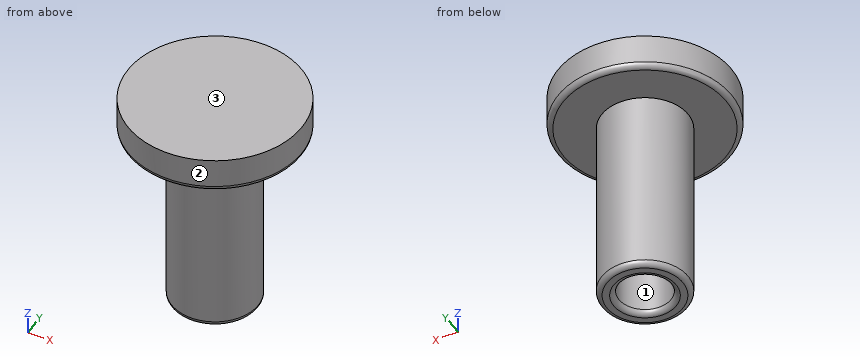
from build123d import *

# Parameters (mm, degrees)
F0_R     = 4.99
F1_DEPTH = 2
F2_R     = 2.485
F3_DEPTH = 11
F4_R     = 1.5
F5_DEPTH = 5
F6_R     = 0.3


with BuildPart() as f1:
    # F0 (on Top) → F1 (new body)
    with BuildSketch(Plane.XY):
        Circle(F0_R)
    extrude(amount=F1_DEPTH)

    # F2 (on face) → F3 (join)
    with BuildSketch(Plane(origin=(0, 0, 0), x_dir=(1, 0, 0), z_dir=(0, 0, -1))):
        Circle(F2_R)
    extrude(amount=F3_DEPTH)

    # F4 (on face) → F5 (cut)
    with BuildSketch(Plane(origin=(0, 0, -11), x_dir=(1, 0, 0), z_dir=(0, 0, -1))):
        Circle(F4_R)
    extrude(amount=-F5_DEPTH, mode=Mode.SUBTRACT)

    # F6
    f6_edges = [f1.edges().sort_by_distance(p)[0] for p in [
        (-2.485, 0, -11),
        (-1.5, 0, -11),
        (-4.99, 0, 0),
    ]]
    fillet(f6_edges, radius=F6_R)


solid = f1.part
Can you work these out from the model? Positions are in its coordinate system, mm. Face numbers are marked on the shaded views. Coordinates: 2 decimals unless noted, no trailing zeros. Loops run counter-clockwise (first coordinate to the right, second up) from the corner with the lowest first, then second, coordinate; pieces in that order, holes last. Notation, with made-up numbers: M 49.25,-31 L 60.25,-31 A20 cw 60.25,-21 Z; hole C 82.25,-32.75 d9. An arc over 180 degrees is marked long. Return JSON: item names as keys, results as strings. Group by question number.
Item 1: I'm going to push flat-ended pins straight in: pin 1 Ø1 at (x, y) = (3, -3) entering from -Z; pin 2 Ø5 at (x, z) = (-1, -2) entering from +Y; pin 3 Ø0.9 at (x, y) = (0, -0.5) entering from -Z; pin 4 Ø2 at (x, z) = (3, -6) entering from -Y. Where does each tip first touch, or does it pass through?
Item 2: Imagine slicing it at A-A (y = 0). Please give me the cut outline in (x, z) (3 decimals).
Item 3: Imagine slicing it at D-D (z = -3.75). Please give me the cut outline in (x, y) (3 decimals).
Item 4: Thinking about a two-plate mould opening in X: for the marked faces 1, 2 and 3, which applies, released by +X, released by -X, zero draft, split by the parting line, or undercut?
Item 5: Imagine slicing it at C-C (z = -7.5). Please give me the cut outline in (x, y) (3 decimals), and give its area (3 significant figures).
Item 6: If I drill on L1, parallel to X at y = 0, z = -9.5 (3 decimals); L2, parallel to Z at x = 3, y = 0, over which ranges is the centre line in solid material (lowest first)? Write a range as from..to.
Verdict:
{
 "1": {"pin 1": "stops at z = 0", "pin 2": "stops at y = 4.99", "pin 3": "stops at z = -6", "pin 4": "stops at y = -1.47"},
 "2": {"outline": "M -4.99,0.3 A0.3 ccw -4.69,0 L -2.485,0 L -2.485,-10.7 A0.3 ccw -2.185,-11 L -1.8,-11 A0.3 ccw -1.5,-10.7 L -1.5,-6 L 1.5,-6 L 1.5,-10.7 A0.3 ccw 1.8,-11 L 2.185,-11 A0.3 ccw 2.485,-10.7 L 2.485,0 L 4.69,0 A0.3 ccw 4.99,0.3 L 4.99,2 L -4.99,2 Z"},
 "3": {"outline": "C 0,0 d4.97"},
 "4": {"face 1": "undercut", "face 2": "split by the parting line", "face 3": "zero draft"},
 "5": {"outline": "C 0,0 d4.97; hole C 0,0 d3", "area": "12.3 mm^2"},
 "6": {"L1": "x = -2.485..-1.5, 1.5..2.485", "L2": "z = 0..2"}
}
